from build123d import *

# Parameters (mm, degrees)
F0_R     = 9.525
F1_DEPTH = 19.05


with BuildPart() as f1:
    # F0 (on Front) → F1 (new body)
    with BuildSketch(Plane.XZ):
        with BuildLine():
            ThreePointArc((10.583333, 11.832526), (14.491826, 6.480942), (15.875, 0))
            ThreePointArc((15.875, 0), (6.480942, -14.491826), (-10.583333, -11.832526))
            ThreePointArc((-10.583333, -11.832526), (95.25, -52.257263), (201.083333, -11.832526))
            ThreePointArc((201.083333, -11.832526), (178.667474, -10.583333), (179.916667, 11.832526))
            ThreePointArc((179.916667, 11.832526), (95.25, -20.507263), (10.583333, 11.832526))
        make_face()
        with BuildLine():
            ThreePointArc((-10.583333, -11.832526), (6.480942, -14.491826), (15.875, 0))
            ThreePointArc((15.875, 0), (14.491826, 6.480942), (10.583333, 11.832526))
            ThreePointArc((10.583333, 11.832526), (-11.832526, 10.583333), (-10.583333, -11.832526))
        make_face()
        Circle(F0_R, mode=Mode.SUBTRACT)
        with BuildLine():
            ThreePointArc((206.375, 0), (196.980942, 14.491826), (179.916667, 11.832526))
            ThreePointArc((179.916667, 11.832526), (178.667474, -10.583333), (201.083333, -11.832526))
            ThreePointArc((201.083333, -11.832526), (204.991826, -6.480942), (206.375, 0))
        make_face()
        with Locations((190.5, 0)):
            Circle(F0_R, mode=Mode.SUBTRACT)
    extrude(amount=F1_DEPTH)


solid = f1.part
Work out the finished part from the listing and answer in its coordinate system (mm). Give positions to 0.01 mm unless a question says otherwise; leave off trailing zeros. Order: outer loops, then holes, each group sorted by start corner. A loop starts at its lowest first (then second) coordinate and runs counter-clockwise, first axis right, second up. Notation, with made-up numbers: (-27, 63.5) - (-21, 63.5) arc R24 ccw to (-21, 84.5) - close; hole circle Ø11 at (48.25, -7.75). An arc over 180 degrees is marked (long way). Answer as CSV lines item,"result". Start each with the question number.
Q1. Given pin 1 Ø10 at (x, y) = (147, -10.5) entering from -Z; pin 2 Ø2 at (y, z) = (-13.5, -8) entering from -X; pin 3 Ø8 at (x, y) = (37, -9.5) entering from -Z; pin 4 Ø11.5 at (x, z) = (0, 0) entering from +Y, each flat-ended and moving along its own axis, determine where each tip first touches the part or whether it passes through.
Q2. The mould has two halves that part along X. Classify faces 1 (the face through (96.5, -9.4, -20.5)), 2 (the face through (180.984, -9.392, 0.419)), 3 (the face through (94, -19.05, -25)), 4 (the face through (93.63, -9.39, -52.25)): +X half, -X half, draft (parallel to the pull), parting line (faces both ways), or undercut.
Q3. The part is cut by section A-A (x = 190.5). Write down the section's boundary in (y, z) (3 decimals), then the cut area to 3 significant figures.
Q4. Find the intervals of material crossed by L1, parallel to X at y = -11.25, z = -6; L2, parallel to Z at x = 0, y = -12.5 (3 decimals); L3, parallel to Z at x = 93.5, y = -14.5, in increasing order. Write a range as [from, to].
Q5. The part is cut by section D-D (x = 28). Write down the section's boundary in (y, z).
Q6. The part is cut by section B-B (y = -13.5). Write down the section's boundary in (x, z) (3 decimals).
Q7. The part is cut by section C-C (z = 7.5). Write down the section's boundary in (x, y), then the cut area to 3 significant figures.
Check result:
1,pin 1,"stops at z = -45.22"
1,pin 2,"stops at x = -14.25"
1,pin 3,"stops at z = -42.7"
1,pin 4,"passes through"
2,face 1,"undercut"
2,face 2,"undercut"
2,face 3,"draft"
2,face 4,"parting line"
3,outline,"(-19.05, -20.507) - (0, -20.507) - (0, -9.525) - (-19.05, -9.525) - close; (-19.05, 9.525) - (0, 9.525) - (0, 15.875) - (-19.05, 15.875) - close"
3,area,"330 mm²"
4,L1,"x = [-14.7, -7.4], [7.4, 36.31], [154.19, 183.1], [197.9, 205.2]"
4,L2,"z = [-20.507, -9.525], [9.525, 15.875]"
4,L3,"z = [-52.25, -20.5]"
5,outline,"(-19.05, -37.31) - (0, -37.31) - (0, -1.24) - (-19.05, -1.24) - close"
6,outline,"(-10.583, -11.833) arc R158.75 ccw to (201.083, -11.833) arc R15.875 ccw to (206.375, 0) arc R15.875 ccw to (179.917, 11.833) arc R127 cw to (10.583, 11.833) arc R15.875 ccw to start; hole circle Ø19.05 at (0, 0); hole circle Ø19.05 at (190.5, 0)"
7,outline,"(-13.99, -19.05) - (-5.87, -19.05) - (-5.87, 0) - (-13.99, 0) - close; (5.87, -19.05) - (15.69, -19.05) - (15.69, 0) - (5.87, 0) - close; (174.81, -19.05) - (184.63, -19.05) - (184.63, 0) - (174.81, 0) - close; (196.37, -19.05) - (204.49, -19.05) - (204.49, 0) - (196.37, 0) - close"
7,area,"684 mm²"
